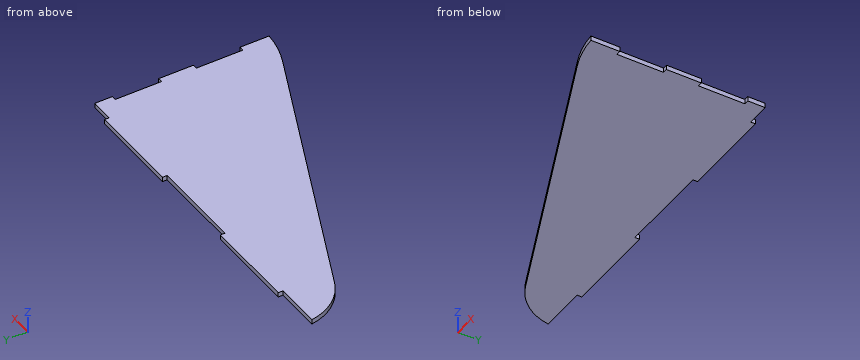
Autodesk Fusion 360 part; units mm, degrees
sketch "Sketch1" plane through (0, 0, 0) normal (0, 0, 1) x (1, 0, 0)
  line L0 (-73.0553, -57.6886) -> (226.9447, -57.6886)
  line L1 (226.9447, 242.3114) -> (-73.0553, 242.3114)
  line L2 (-73.0553, 222.3114) -> (-69.0553, 222.3114)
  line L3 (-69.0553, 222.3114) -> (-69.0553, 142.3114)
  line L4 (-69.0553, 142.3114) -> (-73.0553, 142.3114)
  line L5 (-73.0553, 242.3114) -> (-73.0553, 222.3114)
  line L6 (-73.0553, -17.6886) -> (-69.0553, -17.6886)
  line L7 (-69.0553, -17.6886) -> (-69.0553, 62.3114)
  line L8 (-69.0553, 62.3114) -> (-73.0553, 62.3114)
  line L9 (-73.0553, 142.3114) -> (-73.0553, 62.3114)
  line L10 (-73.0553, -17.6886) -> (-73.0553, -57.6886)
  line L11 (226.9447, 222.3114) -> (222.9447, 222.3114)
  line L12 (222.9447, 222.3114) -> (222.9447, 142.3114)
  line L13 (222.9447, 142.3114) -> (226.9447, 142.3114)
  line L14 (226.9447, 62.3114) -> (222.9447, 62.3114)
  line L15 (222.9447, 62.3114) -> (222.9447, -17.6886)
  line L16 (222.9447, -17.6886) -> (226.9447, -17.6886)
  line L17 (226.9447, -17.6886) -> (226.9447, -57.6886)
  line L18 (226.9447, 142.3114) -> (226.9447, 62.3114)
  line L19 (226.9447, 242.3114) -> (226.9447, 222.3114)
  dimension "d1" = 300
  dimension "d2" = 300
  dimension "d3" = 20
  dimension "d4" = 4
  dimension "d5" = 80
  dimension "d6" = 80
  dimension "d7" = 80
  dimension "d8" = 4
  dimension "d9" = 4
  dimension "d10" = 80
  dimension "d11" = 20
  dimension "d12" = 80
  dimension "d13" = 80
extrude "Extrude1" add sketch "Sketch1" along normal blind 4

Autodesk Fusion 360 part; units mm, degrees
sketch "Sketch1" plane through (0, 0, 0) normal (0, 0, 1) x (1, 0, 0)
  line L0 (-51.5127, 19.8666) -> (-51.5127, 23.8666)
  line L1 (-51.5127, 23.8666) -> (28.4873, 23.8666)
  line L2 (28.4873, 23.8666) -> (28.4873, 19.8666)
  line L3 (-211.5127, 19.8666) -> (-211.5127, 23.8666)
  line L4 (-211.5127, 23.8666) -> (-131.5127, 23.8666)
  line L5 (-131.5127, 23.8666) -> (-131.5127, 19.8666)
  line L6 (48.4873, 4.8666) -> (44.4873, 4.8666)
  line L7 (44.4873, 4.8666) -> (44.4873, -35.1334)
  line L8 (44.4873, -35.1334) -> (48.4873, -35.1334)
  line L9 (48.4873, -65.1334) -> (44.4873, -65.1334)
  line L10 (44.4873, -65.1334) -> (44.4873, -105.1334)
  line L11 (44.4873, -105.1334) -> (48.4873, -105.1334)
  line L12 (-251.5127, 19.8666) -> (-211.5127, 19.8666)
  line L13 (-131.5127, 19.8666) -> (-51.5127, 19.8666)
  line L14 (28.4873, 19.8666) -> (48.4873, 19.8666)
  line L15 (48.4873, 4.8666) -> (48.4873, 6.5368)
  line L16 (48.4873, 6.5368) -> (48.4873, 19.8666)
  line L17 (48.4873, -35.1334) -> (48.4873, -65.1334)
  line L18 (48.4873, -105.1334) -> (48.4873, -130.1334)
  line L19 (17.9193, -122.7788) -> (-223.306, -17.2487)
  arc A0 (-251.5127, 19.8666) -> (-223.306, -17.2487) centre (-204.1197, 26.6083) ccw
  arc A1 (17.9193, -122.7788) -> (48.4873, -130.1334) centre (53.8475, -40.6527) ccw
  dimension "d1" = 300
  dimension "d2" = 150
  dimension "d3" = 4
  dimension "d4" = 4
  dimension "d5" = 80
  dimension "d6" = 80
  dimension "d7" = 20
  dimension "d8" = 80
  dimension "d9" = 4
  dimension "d10" = 4
  dimension "d11" = 40
  dimension "d12" = 40
  dimension "d13" = 30
  dimension "d14" = 15
extrude "Extrude1" add sketch "Sketch1" along normal blind 4
Could you check a few things on this model? Use its own coordinates, in mm. Give positions to 0.01 mm unless a question says otherwise; leave off trailing zeros. Write each loop counter-clockwise with the first axis right and the second up, starting at its lowest first coordinate (ties: lowest second). Pieces come first, ordered by that corner, then holes. Notation, with made-up numbers: (-37.5, 73) -> (-5.5, 73) arc R26 ccw to (-5.5, 108) -> close; hole circle Ø2 at (-8, 8.25). An arc over 180 degrees is marked (long way). Answer as CSV lines item,"result". Start each with the question number.
(1) Please list where these lines run through material, in increasing order: line 1 (Y direction, x = 18, z = 2.05); line 2 (X direction, y = -98, z = 0.85); line 3 (X direction, y = -20.5, z = 3.15).
(2) I'm going to push flat-ended pins straight in: pin 1 Ø1.2 at (x, z) = (47, 1.5) entering from -Y; pin 2 Ø1.5 at (y, z) = (-106, 3.5) entering from -X; pin 3 Ø2 at (y, z) = (-11.5, 2.5) entering from +X. Where does each tip first touch, or does it pass through?
(3) If we section it at C-C, the plane y = -89: Write out the boundary of the cut face in (x, z).
(4) If we section it at B-B, the plane x = -146: Write out the boundary of the cut face in (y, z), and give its area (3 significant figures).
(5) If we section it at A-A, the plane z = 1.45: Write out the boundary of the cut face in (x, y).
Answer list:
1,line 1,"-122.81 to 23.87"
1,line 2,"-38.72 to 44.49"
1,line 3,"-215.87 to 44.49"
2,pin 1,"y = -130.08"
2,pin 2,"x = -22.15"
2,pin 3,"x = 44.49"
3,outline,"(-59.29, 0) -> (44.49, 0) -> (44.49, 4) -> (-59.29, 4) -> close"
4,outline,"(-51.07, 0) -> (23.87, 0) -> (23.87, 4) -> (-51.07, 4) -> close"
4,area,"300 mm^2"
5,outline,"(-251.51, 19.87) arc R47.87 ccw to (-223.31, -17.25) -> (17.92, -122.78) arc R89.64 ccw to (48.49, -130.13) -> (48.49, -105.13) -> (44.49, -105.13) -> (44.49, -65.13) -> (48.49, -65.13) -> (48.49, -35.13) -> (44.49, -35.13) -> (44.49, 4.87) -> (48.49, 4.87) -> (48.49, 19.87) -> (28.49, 19.87) -> (28.49, 23.87) -> (-51.51, 23.87) -> (-51.51, 19.87) -> (-131.51, 19.87) -> (-131.51, 23.87) -> (-211.51, 23.87) -> (-211.51, 19.87) -> close"
